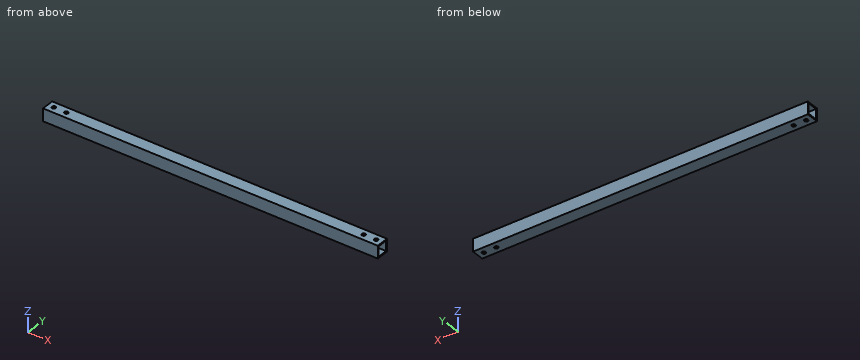
```python
from build123d import *

# Parameters (mm, degrees)
SKETCH1_W           = 20
SKETCH1_H           = 20
SKETCH1_W_2         = 16
SKETCH1_H_2         = 16
BOSS_EXTRUDE1_DEPTH = 268
SKETCH2_R           = 3
CUT_EXTRUDE1_DEPTH  = 269.931217972


with BuildPart() as part:
    # Sketch1 → Boss-Extrude1 (new, symmetric)
    with BuildSketch(Plane(origin=(0, 0, 0), x_dir=(0, 0, -1), z_dir=(1, 0, 0))):
        Rectangle(SKETCH1_W, SKETCH1_H)
        Rectangle(SKETCH1_W_2, SKETCH1_H_2, mode=Mode.SUBTRACT)
    extrude(amount=BOSS_EXTRUDE1_DEPTH, both=True)

    # Sketch2 → Cut-Extrude1 (cut, through all)
    with BuildSketch(Plane.XY.offset(10)):
        with Locations((258, 0)):
            Circle(SKETCH2_R)
        with Locations((238, 0)):
            Circle(SKETCH2_R)
        with Locations((-238, 0)):
            Circle(SKETCH2_R)
        with Locations((-258, 0)):
            Circle(SKETCH2_R)
    extrude(amount=-CUT_EXTRUDE1_DEPTH, mode=Mode.SUBTRACT)


solid = part.part
```
Here's how the part is built. I have some questions about the finished solid (model axes, mm). Round coordinates to 2 decimals unless told otherwise and drop trailing zeros. Write each loop counter-clockwise with the first axis right and the second up, starting at its lowest first coordinate (ties: lowest second). Pieces come first, ordered by that corner, then holes.
Q1. Please list where these lines run through material, in increasing order: probe 1 along Z at (x, y) = (-92.5, 3.75); probe 2 along Y at (x, z) = (258, 8.4).
Q2. Will this pin go through, and if not, where does the flat tip stop? P1, Ø5, axis at y = -2, z = 4.5, coming from the -X side.
Q3. If we section it at A-A on x = 168.5: Write out the boundary of the cut face in (y, z).
Q4. If we section it at B-B on z = -2.75: Write out the boundary of the cut face in (x, y).
Answer below:
1. probe 1: z = -10 to -8, 8 to 10
1. probe 2: y = -10 to -3, 3 to 10
2. P1: passes through
3. outline: (-10, -10) - (10, -10) - (10, 10) - (-10, 10) - close; hole (-8, -8) - (8, -8) - (8, 8) - (-8, 8) - close
4. outline: (-268, -10) - (268, -10) - (268, -8) - (-268, -8) - close; (-268, 8) - (268, 8) - (268, 10) - (-268, 10) - close
